```python
from build123d import *

# Parameters (mm, degrees)
SKETCH2_R          = 1
CUT_EXTRUDE1_DEPTH = 26
SKETCH3_R          = 15
CUT_EXTRUDE2_DEPTH = 22.5


with BuildPart() as part:
    # Sketch1 → Revolve1 (revolve)
    with BuildSketch(Plane.XY):
        with BuildLine():
            Line((-12.5, 15), (-12.5, 0))
            Line((-12.5, 0), (12.5, 0))
            Line((12.5, 0), (12.5, 15))
            Line((12.5, 15), (10, 15))
            ThreePointArc((10, 15), (0, 5), (-10, 15))
            Line((-10, 15), (-12.5, 15))
        make_face()
    revolve(axis=Axis((-12.5, 0, 0), (1, 0, 0)))

    # Sketch2 → Cut-Extrude1 (cut, through all)
    with BuildSketch(Plane(origin=(12.5, 0, 0), x_dir=(0, 0, -1), z_dir=(1, 0, 0))):
        Circle(SKETCH2_R)
    extrude(amount=-CUT_EXTRUDE1_DEPTH, mode=Mode.SUBTRACT)

    # Sketch3 → Cut-Extrude2 (cut)
    with BuildSketch(Plane(origin=(12.5, 0, 0), x_dir=(0, 0, -1), z_dir=(1, 0, 0))):
        Circle(SKETCH3_R)
    extrude(amount=-CUT_EXTRUDE2_DEPTH, mode=Mode.SUBTRACT)


solid = part.part
```
Here's how the part is built. I have some questions about the finished solid (model axes, mm). Give positions to 0.01 mm unless a question says otherwise; leave off trailing zeros. Loops run counter-clockwise (first coordinate to the right, second up) from the corner with the lowest first, then second, coordinate; pieces in that order, holes last. Notation, with made-up numbers: M 32.5,22 L 47.5,22 A13 cw 47.5,47 Z; hole C 58.5,-34.75 d2. An arc over 180 degrees is marked long. Return JSON: item names as keys, results as strings.
Item 1: Thinking about a two-plate mould opening in Z: for faces 1 (the flat face through (-12.5, 0, -3)), 2 (the cylindrical face through (-11, -1, 0)), 3 (the cylindrical face through (-11.268, -14.985, 0.66)), which applies, released by +Z, released by -Z, zero draft, split by the parting line, or undercut?
A:
{"face 1": "zero draft", "face 2": "undercut", "face 3": "split by the parting line"}
Item 2: I'm going to push flat-ended pins straight in: pin 1 Ø1.5 at (x, z) = (-12, 5) entering from +Y; pin 2 Ø1.5 at (x, z) = (-12, 4) entering from -Y. Where does each tip first touch, or does it pass through?
A:
{"pin 1": "stops at y = 14.39", "pin 2": "stops at y = -14.64"}
Item 3: Imagine slicing it at A-A on y = 0. List the corners of the cut face in (x, z) for me.
A:
{"outline": "M -12.5,-15 L -10,-15 L -10,-1 L -12.5,-1 Z; M -12.5,1 L -10,1 L -10,15 L -12.5,15 Z"}
Item 4: Imagine slicing it at D-D on z = -9.5. List the corners of the cut face in (x, y) for me.
A:
{"outline": "M -12.5,-11.61 L -10,-11.61 L -10,11.61 L -12.5,11.61 Z"}
Item 5: Imagine slicing it at C-C on y = -9. List the corners of the cut face in (x, z) for me.
A:
{"outline": "M -12.5,-12 L -10,-12 L -10,12 L -12.5,12 Z"}
Item 6: Please list where these lines run through material, in increasing order: line 1 (Y direction, x = -11.95, z = 0); line 2 (Y direction, x = -11.5, z = 3); line 3 (Z direction, x = -11.9, y = 4).
A:
{"line 1": "y = -15 to -1, 1 to 15", "line 2": "y = -14.7 to 14.7", "line 3": "z = -14.46 to 14.46"}
Item 7: Imagine slicing it at B-B on x = -11.5. List the corners of the cut face in (y, z) for me.
A:
{"outline": "C 0,0 d30; hole C 0,0 d2"}
